Check sheet for the modelled part. Datum: model origin and axes. Units: mm. A direction names the side the tool comes from. Coordinates: 2 decimals unless noted, no trailing zeros. Loops run counter-clockwise (first coordinate to the right, second up) from the corner with the lowest first, then second, coordinate; pieces in that order, holes last. Notation, with made-up numbers: (29.25, 35) - (86.25, 35) arc R27 ccw to (86.25, 70) - close; hole circle Ø6 at (-4, -7). An arc over 180 degrees is marked (long way). Use a Markdown table: item, result. Add a question column.
1) Go/stop test with flat-tipped pins: P1, Ø3, axis at x = 112.5, z = 11.5, coming from the +Y side; P2, Ø14, axis at x = -25.5, y = 21.5, coming from the +Z side; P3, Ø3, axis at y = 7, z = 48.5, coming from the -X side. Record where each tip stops, or that it passes through.
2) Thickness scan on line 1 (Y direction, x = -26, z = 38.5); line 2 (Z direction, x = 8, y = 19); line 3 (Z direction, x = 82.5, y = 27). Record the ranges inside material, lowest first.
3) Sectioned sample at C-C, the plane z = 10. Enter the section's corners in (x, y).
4) Tool access check on faces 4 (the flat face through (84, 27.314, 10)), 5 (the flat face through (-12, -5.759, 32)), 6 (the flat face through (96, 23, 5)). Record the directions out of +Z, -Z, +X, -X, +Y, -Y that give a thin tool (end or side, any length) a straight path to the whole face; none if there is none.
5) Sectioned sample at D-D, the plane z = 35. Enter the section's corners in (x, y).
6) Sectioned sample at A-A, the plane x = -12.5. Enter the section's corners in (y, z).
7) Sectioned sample at B-B, the plane y = 25. Enter the section's corners in (x, z), then the cut area to 3 significant figures.
8) Draft check along X on faces 1 (the flat face through (-12, 23, 0)), 2 (the flat face through (28.374, 23, 10)), 3 (the cylindrical face through (-58.268, 23.096, 46.957)). Enter one of: pulls with the +X half, pulls with the -X half, needs draft (parallel to the pull), parting line crosses it, or undercut.
from build123d import *

# Parameters (mm, degrees)
F0_W      = 127.7185976505
F0_H      = 56.9143816829
F1_DEPTH  = 5
F2_W      = 127.7185976505
F2_H      = 5.2938833833
F2_H_2    = 5.7062916458
F2_W_2    = 112.358585
F2_H_3    = 8.8055357337
F3_DEPTH  = 60
F4_R      = 60
F6_DEPTH  = 46
F7_R      = 8.607172032
F8_DEPTH  = 20
F9_DEPTH  = 25
F10_DEPTH = 50
F5_W      = 67.7185976505
F5_H      = 6.5335953236
F11_DEPTH = 48


with BuildPart() as f1:
    # F0 (on Top) → F1 (new body)
    with BuildSketch(Plane.XY):
        with Locations((-11.5184038877, 22.6980000734)):
            Rectangle(F0_W, F0_H)
    extrude(amount=F1_DEPTH)

    # F2 (on face) → F3 (join)
    with BuildSketch(Plane.XY.offset(5)):
        with Locations((-11.5184038877, 48.5082492232)):
            Rectangle(F2_W, F2_H)
        with Locations((-11.5184038877, -2.9060449451)):
            Rectangle(F2_W, F2_H_2)
        with Locations((84.5533981919, 22.9110382497)):
            Rectangle(F2_W_2, F2_H_3)
    extrude(amount=F3_DEPTH)

    # F4
    f4_edges = [f1.edges().sort_by_distance(p)[0] for p in [
        (-75.377703, 48.508249, 65),
        (-75.377703, -2.906045, 65),
    ]]
    fillet(f4_edges, radius=F4_R)

    # F5 (on face) → F6 (join)
    with BuildSketch(Plane.XZ.offset(-45.8613075316)):
        with BuildLine():
            Line((-15.377702713, 58.4664046764), (-15.377702713, 65))
            ThreePointArc((-15.377702713, 65), (-57.8041095842, 47.4264068712), (-75.377702713, 5))
            Line((-75.377702713, 5), (-70.2792108059, 5))
            ThreePointArc((-70.2792108059, 5), (-53.2827635395, 42.4681154442), (-15.377702713, 58.4664046764))
        make_face()
    extrude(amount=F6_DEPTH)

    # F7 (on face) → F8 (cut)
    with BuildSketch(Plane(origin=(-75.377702713, 0, 0), x_dir=(0, -1, 0), z_dir=(-1, 0, 0))):
        with Locations((-22.6980000734, 20.8706017584)):
            Circle(F7_R)
    extrude(amount=-F8_DEPTH, mode=Mode.SUBTRACT)

    # F7 (on face) → F9 (cut)
    with BuildSketch(Plane(origin=(-75.377702713, 0, 0), x_dir=(0, -1, 0), z_dir=(-1, 0, 0))):
        with Locations((-22.6980000734, 20.8706017584)):
            Circle(F7_R)
    extrude(amount=-F9_DEPTH, mode=Mode.SUBTRACT)

    # F10 (cut): a face of the model
    f10_faces = [f1.faces().sort_by_distance(p)[0] for p in [
        (84.5533981919, 22.9110382497, 65),
    ]]
    extrude(f10_faces, amount=-F10_DEPTH, mode=Mode.SUBTRACT)

    # F5 (on face) → F11 (join)
    with BuildSketch(Plane.XZ.offset(-45.8613075316)):
        with BuildLine():
            Line((-15.377702713, 58.4664046764), (-15.377702713, 65))
            ThreePointArc((-15.377702713, 65), (-57.8041095842, 47.4264068712), (-75.377702713, 5))
            Line((-75.377702713, 5), (-70.2792108059, 5))
            ThreePointArc((-70.2792108059, 5), (-53.2827635395, 42.4681154442), (-15.377702713, 58.4664046764))
        make_face()
        with Locations((18.4815961123, 61.7332023382)):
            Rectangle(F5_W, F5_H)
    extrude(amount=F11_DEPTH)


solid = f1.part
Solved:
| question | item | result |
|---|---|---|
| 1 | P1 | stops at y = 27.31 |
| 1 | P2 | stops at z = 64.92 |
| 1 | P3 | stops at x = -58.23 |
| 2 | line 1 | y = -5.76 to -0.05, 45.86 to 51.16 |
| 2 | line 2 | z = 0 to 5, 58.47 to 65 |
| 2 | line 3 | z = 5 to 15 |
| 3 | outline | (-75.17, -5.76) - (52.34, -5.76) - (52.34, -0.05) - (-69.79, -0.05) - (-69.79, 45.86) - (52.34, 45.86) - (52.34, 51.16) - (-75.17, 51.16) - close; (28.37, 18.51) - (140.73, 18.51) - (140.73, 27.31) - (28.37, 27.31) - close |
| 4 | face 4 | +X |
| 4 | face 5 | +Z, -Z, +X, -X, -Y |
| 4 | face 6 | -Z, +X, +Y, -Y |
| 5 | outline | (-67.34, -5.76) - (52.34, -5.76) - (52.34, -0.05) - (-59.72, -0.05) - (-59.72, 45.86) - (52.34, 45.86) - (52.34, 51.16) - (-67.34, 51.16) - close |
| 6 | outline | (-5.76, 0) - (51.16, 0) - (51.16, 65) - (-5.76, 65) - close; hole (-0.05, 5) - (45.86, 5) - (45.86, 58.47) - (-0.05, 58.47) - close |
| 7 | outline | (-75.38, 0) - (52.34, 0) - (52.34, 5) - (140.73, 5) - (140.73, 15) - (28.37, 15) - (28.37, 5) - (-70.28, 5) arc R56.48 cw to (-15.38, 58.47) - (52.34, 58.47) - (52.34, 65) - (-15.38, 65) arc R60 ccw to (-75.38, 5) - close |
| 7 | area | 2,780 mm2 |
| 8 | face 1 | needs draft |
| 8 | face 2 | undercut |
| 8 | face 3 | pulls with the -X half |
